```python
from build123d import *

# Parameters (mm, degrees)
PAD_DEPTH    = 24
SKETCH_R     = 1.5
POCKET_DEPTH = 5


with BuildPart() as part:
    # Sketch002 → Pad (new body)
    with BuildSketch(Plane.XY):
        with BuildLine():
            Line((10.556671, 23.235573), (12.656862, 21.124397))
            ThreePointArc((12.845641, 20.666956), (12.796592, 20.914388), (12.656862, 21.124397))
            Line((12.845641, 20.666956), (12.845641, -20.493586))
            ThreePointArc((12.691003, -20.868422), (12.805464, -20.696326), (12.845641, -20.493586))
            Line((12.691003, -20.868422), (10.268132, -23.3051))
            ThreePointArc((9.74691, -23.308954), (10.008314, -23.414281), (10.268132, -23.3051))
            Line((9.74691, -23.308954), (6.877814, -20.507596))
            ThreePointArc((6.877814, -20.507596), (6.80996, -20.49473), (6.771762, -20.552268))
            Line((6.771762, -20.552268), (6.771762, -24.661169))
            ThreePointArc((6.771762, -24.661169), (6.832076, -24.80678), (6.977688, -24.867095))
            Line((6.977688, -24.867095), (13.162281, -24.867095))
            ThreePointArc((13.162281, -24.867095), (14.305884, -24.393399), (14.77958, -23.249796))
            Line((14.77958, -23.249796), (14.77958, 22.223828))
            ThreePointArc((14.77958, 22.223828), (14.173704, 23.700512), (12.705269, 24.326117))
            Line((12.705269, 24.326117), (7.387288, 24.397368))
            ThreePointArc((7.387288, 24.397368), (6.844792, 24.178762), (6.619818, 23.638875))
            Line((6.619818, 23.638875), (6.624912, 20.517001))
            ThreePointArc((6.624912, 20.517001), (6.645107, 20.487042), (6.680477, 20.494409))
            Line((6.680477, 20.494409), (9.354538, 23.230274))
            ThreePointArc((10.556671, 23.235573), (9.954496, 23.484367), (9.354538, 23.230274))
        make_face()
    extrude(amount=PAD_DEPTH)

    # Sketch → Pocket (cut)
    with BuildSketch(Plane.YZ.offset(14.77958)):
        with Locations((9.996471, 4.725631)):
            Circle(SKETCH_R)
        with Locations((10.01284, 18.715395)):
            Circle(SKETCH_R)
    extrude(amount=-POCKET_DEPTH, mode=Mode.SUBTRACT)


solid = part.part
```
The model under review builds one solid part; all positions refer to its coordinate system, in mm. A direction names the side the tool comes from. Round coordinates to 2 decimals unless told otherwise and drop trailing zeros. Order: outer loops, then holes, each group sorted by start corner. A loop starts at its lowest first (then second) coordinate and runs counter-clockwise, first axis right, second up.
(1) Take a section at B-B, the plane z = 21.25. State the section outline as (x, y) points.
Working result:
outline: (6.62, 20.52) arc R0.03 ccw to (6.68, 20.49) - (9.35, 23.23) arc R0.84 cw to (10.56, 23.24) - (12.66, 21.12) arc R0.65 cw to (12.85, 20.67) - (12.85, -20.49) arc R0.53 cw to (12.69, -20.87) - (10.27, -23.31) arc R0.37 cw to (9.75, -23.31) - (6.88, -20.51) arc R0.06 ccw to (6.77, -20.55) - (6.77, -24.66) arc R0.21 ccw to (6.98, -24.87) - (13.16, -24.87) arc R1.62 ccw to (14.78, -23.25) - (14.78, 22.22) arc R2.1 ccw to (12.71, 24.33) - (7.39, 24.4) arc R0.76 ccw to (6.62, 23.64) - close
(2) Tool access review of faces 5 (the face through (10, -24.867, 12)), 6 (the face through (11.592, 22.195, 11.832)), 7 (the face through (6.772, -23, 12)): name each direction out of +Z, -Z, +X, -X, +Y, -Y from which nothing blocks a thin tool from reaching the whole face with its end or side.
Working result:
face 5: +Z, -Z, +X, -X, -Y
face 6: +Z, -Z
face 7: +Z, -Z, -X, -Y
(3) Take a section at C-C, the plane x = 11. State the section outline as (y, z) points.
Working result:
outline: (-24.87, 0) - (-22.57, 0) - (-22.57, 24) - (-24.87, 24) - close; (22.79, 0) - (24.35, 0) - (24.35, 24) - (22.79, 24) - close
(4) Take a section at A-A, the plane y = 9.5. State the section outline as (x, z) points (3 decimals).
Working result:
outline: (12.846, 0) - (14.78, 0) - (14.78, 3.31) - (12.846, 3.31) - close; (12.846, 6.141) - (14.78, 6.141) - (14.78, 17.306) - (12.846, 17.306) - close; (12.846, 20.125) - (14.78, 20.125) - (14.78, 24) - (12.846, 24) - close
(5) Mouldability with a two-part tool opening along X and no side actions: class faces 1 (the face through (13, -2, 0)), 2 (the face through (14.78, -1, 12)), 3 (the face through (7.999, 21.843, 11.832)), 4 (the face through (8.332, -21.928, 11.832)) as released by +X, released by -X, zero draft, split by the parting line, or undercut.
Working result:
face 1: zero draft
face 2: released by +X
face 3: undercut
face 4: undercut
(6) Take a section at D-D, the plane y = -22. State the section outline as (x, z) points, plus the area to 3 significant figures.
Working result:
outline: (6.77, 0) - (8.41, 0) - (8.41, 24) - (6.77, 24) - close; (11.57, 0) - (14.78, 0) - (14.78, 24) - (11.57, 24) - close
area: 116 mm2
(7) Wall thickness on L1, parallel to X at y = -9, z = 3.5; L2, parallel to X at y = -22.5, z = 18.25; L3, parallel to Y at x = 9, z = 11.75: over which ranges is each line inside the solid? List them lowest first.
Working result:
L1: x = 12.85 to 14.78
L2: x = 6.77 to 8.92, 11.07 to 14.78
L3: y = -24.87 to -22.58, 22.87 to 24.38
(8) For P1, Ø2, axis at x = 13.5, z = 3.5, coming from the +Y side; P2, Ø1.8, axis at y = 10, z = 4.73, coming from the -X side; P3, Ø1.2, axis at y = -23, z = 16.5, coming from the -X side; P4, Ø10, axis at y = 12, z = 13.5, coming from the -X side, all flat-tipped, find the tip position at first contact; note any pin that passes through.
Working result:
P1: stops at y = 24.33
P2: passes through
P3: stops at x = 6.77
P4: stops at x = 12.85
